Autodesk Fusion 360 part; units mm, degrees
sketch "Esquisse1" plane through (0, 0, 0) normal (0, 0, 1) x (1, 0, 0)
  line L0 (0, 0) -> (150, 0)
  line L1 (150, 0) -> (150, 20)
  line L2 (150, 20) -> (0, 20)
  line L3 (0, 20) -> (0, 0)
  line L4 (0, 20) -> (15, 20)
  line L5 (15, 20) -> (15, 22)
  line L6 (15, 22) -> (0, 22)
  line L7 (0, 22) -> (0, 20)
  line L8 (150, 20) -> (135, 20)
  line L9 (135, 20) -> (135, 22)
  line L10 (135, 22) -> (150, 22)
  line L11 (150, 22) -> (150, 20)
  line L12 (75, 0) -> (75, 20)
  circle A0 centre (10, 3) radius 2.5
  circle A1 centre (140, 3) radius 2.5
  circle A2 centre (85, 3) radius 2
  circle A3 centre (65, 3) radius 2
  dimension "d13" = 150
  dimension "d14" = 20
  dimension "d15" = 5
  dimension "d16" = 5
  dimension "d17" = 4
  dimension "d18" = 4
  dimension "d19" = 10
  dimension "d20" = 10
  dimension "d21" = 10
  dimension "d22" = 10
  dimension "d23" = 3
  dimension "d24" = 3
  dimension "d25" = 3
  dimension "d26" = 3
  dimension "d27" = 2
  dimension "d28" = 15
  dimension "d29" = 15
  dimension "d30" = 2
extrude "Extrusion1" add sketch "Esquisse1" along normal blind 40 contours L2 L4 L5 L6 L7 | L2 L8 L9 L10 L11 makes body 1 at (145, 20, 26.6667) makes body 2 at (10, 22, 26.6667)
extrude "Extrusion2" add sketch "Esquisse1" along normal blind 50 separate body contours A0 | A1 makes body 3 at (12.4876, 2.7511, 16.6667) makes body 4 at (140.6771, 5.4066, 33.3333)
extrude "Extrusion3" add sketch "Esquisse1" along normal blind 30 separate body contours A2 | A3 makes body 5 at (66.3234, 4.4996, 20) makes body 6 at (83.6035, 4.4317, 20)
extrude "Extrusion4" add sketch "Esquisse1" along normal blind 2 contours L0 L2 L3 L4 L12 | L0 L1 L2 L8 L12 bodies 1 2 3 4 5 6
equation "longueur_totale = 150 mm"
equation "largeur_totale = 20 mm"
equation "hauteur_base = 2 mm"
equation "hauteur_plaque_maintien = 40 mm"
equation "hauteur_tube_ext = 50 mm"
equation "hauteur_tube_int = 30 mm"
equation "rayon_tube_ext = 5 mm"
equation "rayon_tube_int = 4 mm"
equation "longueur_plaque_maintien = 15 mm"
equation "largeur_plaque_maintien = 2 mm"
equation "ecart_tube_int_centre = 10 mm"
equation "d13 = longueur_totale"
equation "d14 = largeur_totale"
equation "d15 = rayon_tube_ext"
equation "d16 = rayon_tube_ext"
equation "d17 = rayon_tube_int"
equation "d18 = rayon_tube_int"
equation "d19 = Linear Dimension-4"
equation "d20 = Linear Dimension-5"
equation "d21 = ecart_tube_int_centre"
equation "d22 = ecart_tube_int_centre"
equation "d24 = d23"
equation "d25 = d23"
equation "d26 = d23"
equation "d27 = largeur_plaque_maintien"
equation "d28 = longueur_plaque_maintien"
equation "d29 = longueur_plaque_maintien"
equation "d30 = largeur_plaque_maintien"
equation "d31 = hauteur_plaque_maintien"
equation "d33 = hauteur_tube_ext"
equation "d35 = hauteur_tube_int"
equation "d37 = hauteur_base"
Here's how the part is built. I have some questions about the finished solid (model axes, mm). A direction names the side the tool comes from. Coordinates: 2 decimals unless noted, no trailing zeros. Order: outer loops, then holes, each group sorted by start corner. A loop starts at its lowest first (then second) coordinate and runs counter-clockwise, first axis right, second up. Notation, with made-up numbers: (44.25, -29) - (101.25, -29) arc R24 cw to (101.25, -13) - close; hole circle Ø3 at (57.25, 64). An arc over 180 degrees is marked (long way). One line per question, with ' | ' between items.
(1) Suppose I cut it at B-B on x = 140. List the corners of the cut face in (y, z) for me.
Report:
outline: (0, 0) - (22, 0) - (22, 40) - (20, 40) - (20, 2) - (5.5, 2) - (5.5, 50) - (0.5, 50) - (0.5, 2) - (0, 2) - close
(2) If we mould it in two halves opening along Y, with no side actions, what happens to faces 6 (the flat face through (85, 3, 30)), 7 (the flat face through (8, 20, 21)), 8 (the cylindrical face through (63, 3, 16))? For each: pulls with the +Y half, pulls with the -Y half, needs draft (parallel to the pull), parting line crosses it, or undercut.
Report:
face 6: needs draft | face 7: undercut | face 8: parting line crosses it
(3) Suppose I cut it at A-A on z = 33.5. List the corners of the cut face in (x, y) for me.
Report:
outline: (0, 20) - (15, 20) - (15, 22) - (0, 22) - close; circle Ø5 at (10, 3); (135, 20) - (150, 20) - (150, 22) - (135, 22) - close; circle Ø5 at (140, 3)
(4) Suppose I cut it at C-C on y = 3. List the corners of the cut face in (x, z) for me, and give its area (3 significant figures).
Report:
outline: (0, 0) - (150, 0) - (150, 2) - (142.5, 2) - (142.5, 50) - (137.5, 50) - (137.5, 2) - (87, 2) - (87, 30) - (83, 30) - (83, 2) - (67, 2) - (67, 30) - (63, 30) - (63, 2) - (12.5, 2) - (12.5, 50) - (7.5, 50) - (7.5, 2) - (0, 2) - close | area: 1,000 mm2
(5) Suppose I cut it at D-D on x = 65. List the corners of the cut face in (y, z) for me.
Report:
outline: (0, 0) - (20, 0) - (20, 2) - (5, 2) - (5, 30) - (1, 30) - (1, 2) - (0, 2) - close
(6) If I drill on L1, parallel to X at y = 4.75, z = 4; L2, parallel to X at y = 20.75, z = 4; L3, parallel to Z at x = 136, y = 4.5, over which ranges is the centre line in solid material (lowest first)?
Report:
L1: x = 8.21 to 11.79, 64.03 to 65.97, 84.03 to 85.97, 138.21 to 141.79 | L2: x = 0 to 15, 135 to 150 | L3: z = 0 to 2
(7) For faces 1 (the flat face through (150, 21, 15)), 2 (the flat face through (65, 3, 30)), 3 (the flat face through (140, 3, 50)), 4 (the cylindrical face through (9.46, 5.44, 25.66)), 5 (the flat face through (143, 20, 21)), which set-ups out of +Z, -Z, +X, -X, +Y, -Y let a thin tool reach every point of the face, with its end or its side?
Report:
face 1: +Z, -Z, +X, +Y, -Y | face 2: +Z, +Y, -Y | face 3: +Z, +X, -X, +Y, -Y | face 4: +Z | face 5: +Z, +X, -X
(8) Will these pins go through, and if not, where does the flat tip stop? pin 1 (1.5 mm diameter, centred on x = 118, y = 7.5, fed in from +Z); pin 2 (0.6 mm diameter, centred on x = 10.5, y = 21.5, fed in from +Z); pin 3 (4.5 mm diameter, centred on x = 84, y = 3, fed in from +Z).
Report:
pin 1: stops at z = 2 | pin 2: stops at z = 40 | pin 3: stops at z = 30
